Could you check a few things on this model? Use its own coordinates, in mm. Coordinates: 2 decimals unless noted, no trailing zeros. Write each loop counter-clockwise with the first axis right and the second up, starting at its lowest first coordinate (ties: lowest second). Pieces come first, ordered by that corner, then holes.
Item 1: If I drill on probe 1 along Y at (x, z) = (0.5, 2.2); probe 2 along X at (y, z) = (-180, 2.7); probe 3 along X at (y, z) = (2, 0.25), over which ranges is the centre line in solid material (lowest first)?
Item 2: I want a section at C-C on x = -164. Please give me the cut outline in (y, z).
Item 3: I want a section at B-B on y = -181. Please give me the cut outline in (x, z).
Item 4: I want a section at A-A on x = 0. Please give me the cut outline in (y, z), then the cut area to 3 significant figures.
Item 5: I want a section at D-D on z = 2.45. State how many separate pieces and enclosed holes the cut face has, then the cut area to 3 significant figures.
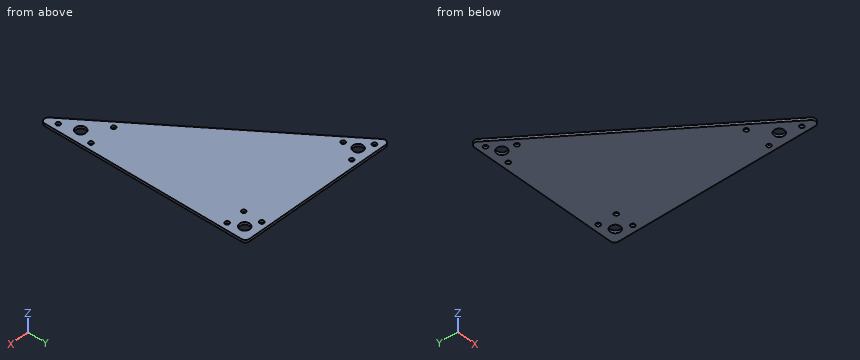
from build123d import *

# Parameters (mm, degrees)
SKETCH_2_R      = 6.05
SKETCH_2_R_2    = 2.55
SKETCH_2_R_3    = 2.6
EXTRUDE_1_DEPTH = 3
FILLET_1_R      = 5


with BuildPart() as part:
    # 草图2 → 凸台-拉伸1 (new body)
    with BuildSketch(Plane.XY):
        Polygon((-180, 15), (15, 15), (15, -245), align=None)
        Circle(SKETCH_2_R, mode=Mode.SUBTRACT)
        with Locations((-150, 0)):
            Circle(SKETCH_2_R, mode=Mode.SUBTRACT)
        with Locations((0, -200)):
            Circle(SKETCH_2_R, mode=Mode.SUBTRACT)
        with Locations((-164, 7)):
            Circle(SKETCH_2_R_2, mode=Mode.SUBTRACT)
        with Locations((-134, 7)):
            Circle(SKETCH_2_R_2, mode=Mode.SUBTRACT)
        with Locations((-147.04893552, -15.601419306)):
            Circle(SKETCH_2_R_2, mode=Mode.SUBTRACT)
        with Locations((-15, 7)):
            Circle(SKETCH_2_R_3, mode=Mode.SUBTRACT)
        with Locations((7, -15)):
            Circle(SKETCH_2_R_2, mode=Mode.SUBTRACT)
        with Locations((7, -221)):
            Circle(SKETCH_2_R_3, mode=Mode.SUBTRACT)
        with Locations((-23, -181)):
            Circle(SKETCH_2_R_3, mode=Mode.SUBTRACT)
        with Locations((7, -181)):
            Circle(SKETCH_2_R_3, mode=Mode.SUBTRACT)
        with Locations((-15, -15)):
            Circle(SKETCH_2_R_2, mode=Mode.SUBTRACT)
    extrude(amount=EXTRUDE_1_DEPTH)

    # 圆角1
    fillet_1_edges = [part.edges().sort_by_distance(p)[0] for p in [
        (-180, 15, 1.5),
        (15, 15, 1.5),
        (15, -245, 1.5),
    ]]
    fillet(fillet_1_edges, radius=FILLET_1_R)


solid = part.part
Response values:
1. probe 1: y = -225.67 to -206.03, -193.97 to -6.03, 6.03 to 15
1. probe 2: x = -33.75 to -25.4, -20.6 to 4.6, 9.4 to 15
1. probe 3: x = -170.25 to -155.71, -144.29 to -5.71, 5.71 to 15
2. outline: (-6.33, 0) - (4.45, 0) - (4.45, 3) - (-6.33, 3) - close; (9.55, 0) - (15, 0) - (15, 3) - (9.55, 3) - close
3. outline: (-33, 0) - (-25.6, 0) - (-25.6, 3) - (-33, 3) - close; (-20.4, 0) - (4.4, 0) - (4.4, 3) - (-20.4, 3) - close; (9.6, 0) - (15, 0) - (15, 3) - (9.6, 3) - close
4. outline: (-225, 0) - (-206.05, 0) - (-206.05, 3) - (-225, 3) - close; (-193.95, 0) - (-6.05, 0) - (-6.05, 3) - (-193.95, 3) - close; (6.05, 0) - (15, 0) - (15, 3) - (6.05, 3) - close
4. area: 647 mm2
5. separate pieces: 1
5. enclosed holes: 12
5. area: 24,700 mm2
